Can you work these out from the model? Positions are in its coordinate system, mm. A direction names the side the tool comes from. Give positions to 0.01 mm unless a question says otherwise; leave off trailing zeros. Order: outer loops, then holes, each group sorted by start corner. A loop starts at its lowest first (then second) coordinate and runs counter-clockwise, first axis right, second up. Notation, with made-up numbers: M 50.5,-6.75 L 103.5,-6.75 A16 ccw 103.5,2.25 Z; hole C -33,-16 d10. An arc over 180 degrees is marked long. Use a Markdown table: item, result. Add a question column.
from build123d import *

# Parameters (mm, degrees)
SKETCH_1_R          = 10
EXTRUDE_1_DEPTH     = 1
SKETCH_2_R          = 4.5
EXTRUDE_2_DEPTH     = 1
SKETCH_3_R          = 2.5
CUT_EXTRUDE_1_DEPTH = 15.282856857
SKETCH_4_R          = 0.5
CUT_EXTRUDE_2_DEPTH = 15.282856857


with BuildPart() as part:
    # 草图1 → 凸台-拉伸1 (new body)
    with BuildSketch(Plane.XY):
        Circle(SKETCH_1_R)
    extrude(amount=EXTRUDE_1_DEPTH)

    # 草图2 → 凸台-拉伸2 (add)
    with BuildSketch(Plane.XY.offset(1)):
        Circle(SKETCH_2_R)
    extrude(amount=EXTRUDE_2_DEPTH)

    # 草图3 → 切除-拉伸1 (cut, through all)
    with BuildSketch(Plane.XY.offset(2)):
        Circle(SKETCH_3_R)
    extrude(amount=-CUT_EXTRUDE_1_DEPTH, mode=Mode.SUBTRACT)

    # 草图4 → 切除-拉伸2 (cut, through all)
    with BuildSketch(Plane(origin=(0, 0, 0), x_dir=(-1, 0, 0), z_dir=(0, 0, -1))):
        with Locations((0, 8)):
            Circle(SKETCH_4_R)
        with Locations((8, 0)):
            Circle(SKETCH_4_R)
        with Locations((0, -8)):
            Circle(SKETCH_4_R)
        with Locations((-8, 0)):
            Circle(SKETCH_4_R)
    extrude(amount=-CUT_EXTRUDE_2_DEPTH, mode=Mode.SUBTRACT)


solid = part.part
1. If we section it at C-C, the plane y = 0: List the corners of the cut face in (x, z) for me, then the cut area to 3 significant figures.
2. We'd pull the mould along Y, two halves only. Please class faces 3 (the face through (0.108, 7.512, 0.493)), 4 (the face through (2, -2, 2)), 5 (the face through (-0.59, 4.46, 1.49)), 6 (the face through (0.108, -8.488, 0.493)): +Y half, -Y half, draft (parallel to the pull), parting line (faces both ways), or undercut.
3. If we section it at A-A, the plane y = 8: List the corners of the cut face in (x, z) for me, then the cut area to 3 significant figures.
4. If we section it at D-D, the plane z = 0.5: List the corners of the cut face in (x, y) for me, then the cut area to 3 significant figures.
5. On a 3-axis mill with a long thin cutter (end or side, diameter ignored), from which of +Z, -Z, +X, -X, +Y, -Y can I reach the whole of each face in a straight line? I mean faces 1 (the face through (-0.54, -2.44, 1.01)), 2 (the face through (4.3, -2.1, 1)). Say none if no direction works.
6. I need wall thicknesses on L1, parallel to Y at x = 0, z = 0.3; L2, parallel to Z at x = -2, y = -6.5; L3, parallel to X at y = 2, z = 1.65. Which ranges of each line are inside material? Lowest first, please. Write a range as [from, to].
7. Will these pins go through, and if not, where does the flat tip stop? pin 1 (1 mm diameter, centred on y = 1.5, z = 0, fed in from -X); pin 2 (1 mm diameter, centred on y = 6, z = 0.5, fed in from -X); pin 3 (1.5 mm diameter, centred on x = 7, y = 0, fed in from +Z).
Geometry results:
| question | item | result |
|---|---|---|
| 1 | outline | M -10,0 L -8.5,0 L -8.5,1 L -10,1 Z; M -7.5,0 L -2.5,0 L -2.5,2 L -4.5,2 L -4.5,1 L -7.5,1 Z; M 2.5,0 L 7.5,0 L 7.5,1 L 4.5,1 L 4.5,2 L 2.5,2 Z; M 8.5,0 L 10,0 L 10,1 L 8.5,1 Z |
| 1 | area | 17.0 mm^2 |
| 2 | face 3 | undercut |
| 2 | face 4 | draft |
| 2 | face 5 | parting line |
| 2 | face 6 | undercut |
| 3 | outline | M -6,0 L -0.5,0 L -0.5,1 L -6,1 Z; M 0.5,0 L 6,0 L 6,1 L 0.5,1 Z |
| 3 | area | 11.0 mm^2 |
| 4 | outline | C 0,0 d20; hole C -8,0 d1; hole C 0,0 d5; hole C 0,-8 d1; hole C 0,8 d1; hole C 8,0 d1 |
| 4 | area | 291 mm^2 |
| 5 | face 1 | +Z, -Z |
| 5 | face 2 | +Z |
| 6 | L1 | y = [-10, -8.5], [-7.5, -2.5], [2.5, 7.5], [8.5, 10] |
| 6 | L2 | z = [0, 1] |
| 6 | L3 | x = [-4.03, -1.5], [1.5, 4.03] |
| 7 | pin 1 | stops at x = -9.95 |
| 7 | pin 2 | stops at x = -8.35 |
| 7 | pin 3 | stops at z = 1 |
